Read the model definition and answer for the solid it produces. Units are mm, in the model's axes. A direction names the side the tool comes from. Coordinates: 2 decimals unless noted, no trailing zeros. Write each loop counter-clockwise with the first axis right and the second up, starting at its lowest first coordinate (ties: lowest second). Pieces come first, ordered by that corner, then holes. Notation, with made-up numbers: (60, -10) -> (71, -10) arc R33 cw to (71, 24) -> close; hole circle Ø2 at (-10, 82.25). An arc over 180 degrees is marked (long way). Answer in a Markdown table with one row per item. Add a question column.
Item 1: Given pin 1 Ø8.5 at (x, y) = (76.5, 11) entering from -Z; pin 2 Ø8 at (x, z) = (44, 56) entering from -Y; pin 3 Ø15 at (y, z) = (7, -4.5) entering from -X (3 decimals), each flat-ended and moving along its own axis, determine where each tip first touches the part or whether it passes through.
Item 2: Section A-A on y = -34.5 is taken. Write down the section's boundary in (x, z) (3 decimals).
Item 3: Which of the six approach directions +Z, -Z, +X, -X, +Y, -Y give full straight-line access (tool end or side, diameter ignored) to faces 1 (the face through (60, 2, 42.875)), 2 (the face through (-4, 7.938, 30)), 3 (the face through (86, 0, 38.1))?
Item 4: Straight lines are drawn through the part: line 1 (Z direction, x = -23.5, y = -31.5) (3 decimals); line 2 (Y direction, x = 68, z = 51); line 3 (Y direction, x = 18, z = 30). For each, find the intervals that lie inside material, in ascending order. Write a range as from..to.
```python
from build123d import *

# Parameters (mm, degrees)
F1_DEPTH = 63.5
F0_W     = 25.4
F0_H     = 19.05
F2_DEPTH = 25.4
F4_R     = 6.35
F5_DEPTH = 7.9375


with BuildPart() as f1:
    # F0 (on Front) → F1 (new body, symmetric)
    with BuildSketch(Plane.XZ):
        Polygon((41.275, -9.525), (41.275, 9.525), (22.225, 9.525), (-41.275, 9.525), (-41.275, -9.525), align=None)
    extrude(amount=F1_DEPTH, both=True)

    # F0 (on Front) → F2 (join, symmetric)
    with BuildSketch(Plane.XZ):
        with BuildLine():
            Line((22.225, 9.525), (41.275, 9.525))
            Line((41.275, 9.525), (41.275, 27.0002))
            ThreePointArc((41.275, 27.0002), (45.9246798487, 38.2255201513), (57.15, 42.8752))
            Line((57.15, 42.8752), (60.325, 42.8752))
            Line((60.325, 42.8752), (60.325, 61.9252))
            Line((60.325, 61.9252), (57.15, 61.9252))
            add(Edge.make_bspline(
                [(56.7889636958, 61.9233338483), (56.9093507324, 61.9240660215), (57.0296965137, 61.9246880569), (57.15, 61.9252)],
                knots=[111.215608545, 111.215608545, 111.215608545, 111.215608545, 111.5045361635, 111.5045361635, 111.5045361635, 111.5045361635], degree=3))
            ThreePointArc((56.7889636958, 61.9233338483), (32.3269782468, 51.567927124), (22.225, 27.0002))
            Line((22.225, 27.0002), (22.225, 9.525))
        make_face()
        with Locations((73.025, 52.4002)):
            Rectangle(F0_W, F0_H)
    extrude(amount=F2_DEPTH, both=True)

    # F0 (on Front) → F3 (revolve)
    with BuildSketch(Plane.XZ):
        Polygon((85.725, 61.9252), (85.725, 42.8752), (85.725, 38.1), (111.125, 38.1), (111.125, 66.675), (85.725, 66.675), align=None)
    revolve(axis=Axis((85.725, 0, 52.3875), (0, 0, 1)))

    # F4
    f4_edges = [f1.edges().sort_by_distance(p)[0] for p in [
        (41.275, -63.5, 0),
        (-41.275, -63.5, 0),
        (41.275, 63.5, 0),
        (-41.275, 63.5, 0),
    ]]
    fillet(f4_edges, radius=F4_R)

    # F0 (on Front) → F5 (join, symmetric)
    with BuildSketch(Plane.XZ):
        with BuildLine():
            Line((-41.275, 9.525), (22.225, 9.525))
            Line((22.225, 9.525), (22.225, 27.0002))
            ThreePointArc((22.225, 27.0002), (32.3269782468, 51.567927124), (56.7889636958, 61.9233338483))
            add(Edge.make_bspline(
                [(-41.275, 9.525), (-42.0038243378, 45.0408061819), (10.4489232116, 61.6415017024), (56.7889636958, 61.9233338483)],
                knots=[0, 0, 0, 0, 111.215608545, 111.215608545, 111.215608545, 111.215608545], degree=3))
        make_face()
    extrude(amount=F5_DEPTH, both=True)


solid = f1.part
```
Results below:
| question | item | result |
|---|---|---|
| 1 | pin 1 | stops at z = 38.1 |
| 1 | pin 2 | stops at y = -25.4 |
| 1 | pin 3 | stops at x = -41.275 |
| 2 | outline | (-41.275, -9.525) -> (41.275, -9.525) -> (41.275, 9.525) -> (-41.275, 9.525) -> close |
| 3 | face 1 | -Z |
| 3 | face 2 | +Z, -X, +Y |
| 3 | face 3 | -Z, +X, +Y, -Y |
| 4 | line 1 | z = -9.525..9.525 |
| 4 | line 2 | y = -25.4..25.4 |
| 4 | line 3 | y = -7.94..7.94 |
